Model file for the job. Use its own axes, mm. Face numbers are marked on the shaded views. Coordinates: 2 decimals unless noted, no trailing zeros. Loops run counter-clockwise (first coordinate to the right, second up) from the corner with the lowest first, then second, coordinate; pieces in that order, holes last.
from build123d import *

# Parameters (mm, degrees)
SKETCH1_R           = 5.95
BOSS_EXTRUDE1_DEPTH = 9.6
SKETCH2_R           = 1.241958451
CUT_EXTRUDE1_DEPTH  = 2
SKETCH3_R           = 0.425
BOSS_EXTRUDE2_DEPTH = 3


with BuildPart() as part:
    # Sketch1 → Boss-Extrude1 (new body)
    with BuildSketch(Plane.XY):
        Circle(SKETCH1_R)
    extrude(amount=BOSS_EXTRUDE1_DEPTH)

    # Sketch2 → Cut-Extrude1 (cut)
    with BuildSketch(Plane.XY.offset(9.6)):
        Circle(SKETCH2_R)
    extrude(amount=-CUT_EXTRUDE1_DEPTH, mode=Mode.SUBTRACT)

    # Sketch3 → Boss-Extrude2 (add)
    with BuildSketch(Plane(origin=(0, 0, 0), x_dir=(-1, 0, 0), z_dir=(0, 0, -1))):
        with Locations((-3.75, 0)):
            Circle(SKETCH3_R)
        with Locations((3.75, 0)):
            Circle(SKETCH3_R)
    extrude(amount=BOSS_EXTRUDE2_DEPTH)


solid = part.part
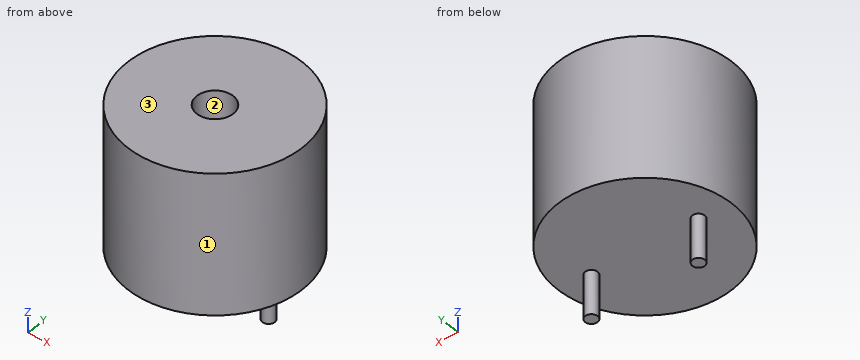
Q1. Slice it at B-B (y = 0). List the corners of the cut face in (x, z) (3 decimals), and give its area (3 significant figures).
Answers:
outline: (-5.95, 0) - (-4.175, 0) - (-4.175, -3) - (-3.325, -3) - (-3.325, 0) - (3.325, 0) - (3.325, -3) - (4.175, -3) - (4.175, 0) - (5.95, 0) - (5.95, 9.6) - (1.242, 9.6) - (1.242, 7.6) - (-1.242, 7.6) - (-1.242, 9.6) - (-5.95, 9.6) - close
area: 114 mm2
Q2. Slice it at C-C (z = 4.5). List the corners of the cut face in (x, y).
Answers:
outline: circle Ø11.9 at (0, 0)
Q3. Slice it at D-D (z = 8.5). List the corners of the cut face in (x, y), and give its area (3 significant figures).
Answers:
outline: circle Ø11.9 at (0, 0); hole circle Ø2.48 at (0, 0)
area: 106 mm2
Q4. Drill centre lines: line 1 (Y direction, x = 0, z = 8.05); line 2 (Z direction, x = -4.75, y = 0.5); line 3 (Z direction, x = 0.5, y = 0.75). Where is each one in solid material? Low to high.
Answers:
line 1: y = -5.95 to -1.24, 1.24 to 5.95
line 2: z = 0 to 9.6
line 3: z = 0 to 7.6
Q5. Slice it at A-A (x = 0). List the corners of the cut face in (y, z), and give its area (3 significant figures).
Answers:
outline: (-5.95, 0) - (5.95, 0) - (5.95, 9.6) - (1.24, 9.6) - (1.24, 7.6) - (-1.24, 7.6) - (-1.24, 9.6) - (-5.95, 9.6) - close
area: 109 mm2
Q6. Flat gauge pins, fed straight in: P1, Ø5, axis at x = 4.5, y = -4, coming from the -Z side; P2, Ø1, axis at x = -1, z = 3, coming from the +Y side; P3, Ø6, axis at x = -4.5, z = 7.5, coming from the +Y side. Where does each tip first touch, or does it go through?
Answers:
P1: stops at z = 0
P2: stops at y = 5.93
P3: stops at y = 5.76
Q7. Mould opens along X. For the marked faces 1, 2 and 3 say: +X half, -X half, draft (parallel to the pull), parting line (faces both ways), or undercut.
Answers:
face 1: parting line
face 2: undercut
face 3: draft
